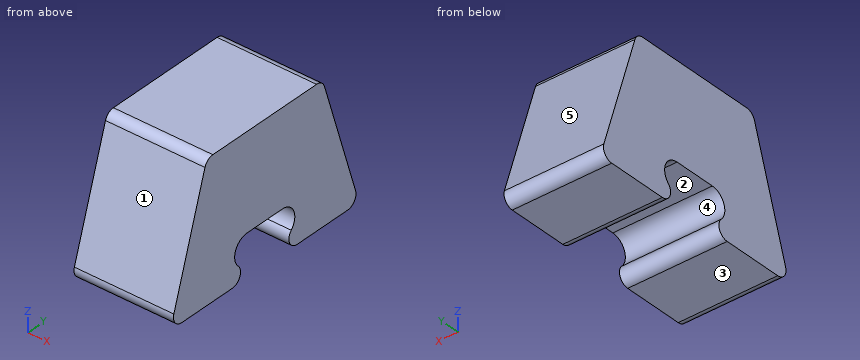
from build123d import *

# Parameters (mm, degrees)
BOSS_EXTRUDE1_DEPTH      = 1
BOSS_EXTRUDE1_DEPTH_BACK = 3


with BuildPart() as part:
    # Sketch3 → Boss-Extrude1 (new, two sides: drawn at the far end of the back side and taken through both)
    with BuildSketch(Plane.YZ.offset(-BOSS_EXTRUDE1_DEPTH_BACK)):
        with BuildLine():
            Line((-4, 5.4), (-1.56416825, 5.4))
            ThreePointArc((-1.56416825, 5.4), (-1.195386471, 5.645080666), (-1.278511113, 6.08))
            ThreePointArc((-1.278511113, 6.08), (-1.403198074, 6.732379001), (-0.850025407, 7.1))
            Line((-0.850025407, 7.1), (0.850025407, 7.1))
            ThreePointArc((0.850025407, 7.1), (1.403198074, 6.732379001), (1.278511113, 6.08))
            ThreePointArc((1.278511113, 6.08), (1.195386471, 5.645080666), (1.56416825, 5.4))
            Line((1.56416825, 5.4), (4, 5.4))
            ThreePointArc((4, 5.4), (4.322991043, 5.564040711), (4.381063684, 5.92161607))
            Line((4.381063684, 5.92161607), (2.881063684, 10.62161607))
            ThreePointArc((2.881063684, 10.62161607), (2.735959289, 10.822991043), (2.5, 10.9))
            Line((2.5, 10.9), (-2.5, 10.9))
            ThreePointArc((-2.5, 10.9), (-2.735959289, 10.822991043), (-2.881063684, 10.62161607))
            Line((-2.881063684, 10.62161607), (-4.381063684, 5.92161607))
            ThreePointArc((-4.381063684, 5.92161607), (-4.322991043, 5.564040711), (-4, 5.4))
        make_face()
    extrude(amount=BOSS_EXTRUDE1_DEPTH + BOSS_EXTRUDE1_DEPTH_BACK)


solid = part.part
Build history of the part. All positions in model axes, mm. Face numbers are marked on the shaded views. A direction names the side the tool comes from. Coordinates: 2 decimals unless noted, no trailing zeros. Write each loop counter-clockwise with the first axis right and the second up, starting at its lowest first coordinate (ties: lowest second). Pieces come first, ordered by that corner, then holes. Notation, with made-up numbers: (4, 79) -> (49, 79) arc R22 ccw to (49, 95) -> close; hole circle Ø7 at (45.5, -37.5). An arc over 180 degrees is marked (long way). Use CSV: the item, a comma, the result in double quotes. Start each with the question number.
Q1. Cut at C-C, the plane y = 0.25. List the corners of the cut face in (x, z).
Q2. Drill centre lines: probe 1 along Z at (x, y) = (-2.2, -0.75); probe 2 along Y at (x, z) = (-2, 6.95); probe 3 along Y at (x, z) = (-2.25, 10.5). Where is each one in solid material? Low to high.
Q3. Flat gauge pins, fed straight in: pin 1 Ø1 at (x, z) = (-2.5, 10.5) entering from +Y; pin 2 Ø1.9 at (x, y) = (-0.5, 0) entering from -Z. Where does each tip first touch, or does it go through?
Q4. Pull direction Y, two halves, no side cores. Call the marked faces 1, 2 and 3: released by +Y, released by -Y, zero draft, split by the parting line, or undercut.
Q5. Cut at A-A, the plane z = 6.35. List the corners of the cut face in (x, y).
Q6. Cut at D-D, the plane z = 9.5. List the corners of the cut face in (x, y).
Q7. Cut at B-B, the plane x = -1.1. List the corners of the cut face in (y, z), then the cut area to 3 significant figures.
Q8. 3-axis set-ups, long thin cutter, end or side, ignore diameter. For the marked faces 4 and 5: which of +Z, -Z, +X, -X, +Y, -Y reach the whole face in a straight line?
Checked values:
1,outline,"(-3, 7.1) -> (1, 7.1) -> (1, 10.9) -> (-3, 10.9) -> close"
2,probe 1,"z = 7.1 to 10.9"
2,probe 2,"y = -4.05 to -1.25, 1.25 to 4.05"
2,probe 3,"y = -2.92 to 2.92"
3,pin 1,"stops at y = 3.08"
3,pin 2,"stops at z = 7.09"
4,face 1,"released by -Y"
4,face 2,"undercut"
4,face 3,"zero draft"
5,outline,"(-3, -4.24) -> (1, -4.24) -> (1, -1.43) -> (-3, -1.43) -> close; (-3, 1.43) -> (1, 1.43) -> (1, 4.24) -> (-3, 4.24) -> close"
6,outline,"(-3, -3.24) -> (1, -3.24) -> (1, 3.24) -> (-3, 3.24) -> close"
7,outline,"(-4.38, 5.92) arc R0.4 ccw to (-4, 5.4) -> (-1.56, 5.4) arc R0.4 ccw to (-1.28, 6.08) arc R0.6 cw to (-0.85, 7.1) -> (0.85, 7.1) arc R0.6 cw to (1.28, 6.08) arc R0.4 ccw to (1.56, 5.4) -> (4, 5.4) arc R0.4 ccw to (4.38, 5.92) -> (2.88, 10.62) arc R0.4 ccw to (2.5, 10.9) -> (-2.5, 10.9) arc R0.4 ccw to (-2.88, 10.62) -> close"
7,area,"35.8 mm²"
8,face 4,"+X, -X"
8,face 5,"+Z, +X, -X, +Y"
